Job drawing, mm, ordinate dimensions from the low corner. One solid piece. A direction names the side the tool comes from. Coordinates: 2 decimals unless noted, no trailing zeros. Order: outer loops, then holes, each group sorted by start corner. A loop starts at its lowest first (then second) coordinate and runs counter-clockwise, first axis right, second up. Notation, with made-up numbers: (-33, -11) -> (-16, -11) arc R26 ccw to (-16, 24) -> close; hole circle Ø10 at (-8.75, 29.5). An arc over 180 degrees is marked (long way). Use CSV: the item, a comma, the result in double quotes. Start each with the question number.
(1) Pin check, flat tips, straight feed: pin 1 Ø2 at (x, z) = (8, 4) entering from +Y; pin 2 Ø4 at (x, y) = (6, 11) entering from +Z. Stop position of each tip, or through.
(2) Cut at D-D on y = 3.25. Write the cut outline in (x, z).
(3) Cut at B-B on y = 6.35. Write the cut outline in (x, z).
(4) Probe L1, parallel to Z at x = 5, y = 6.35; L2, parallel to Y at x = 2.75, z = 2.25; L3, parallel to Z at x = 6, y = 1.75. List the from-to ranges inside material, lowest first.
(5) Pull direction Z, two halves, no side cores. Call the marked faces 6, 7 and 8: pulls with the +Z half, pulls with the -Z half, needs draft (parallel to the pull), parting line crosses it, or undercut.
(6) Cut at C-C on z = 1.9. Write the cut outline in (x, y), plus the area to 3 significant figures.
(7) Tool access for the marked faces 1, 2, 3, 4 and 5: list every direction of +Z, -Z, +X, -X, +Y, -Y with a clear straight run to the whole face (end or side of a thin tool).
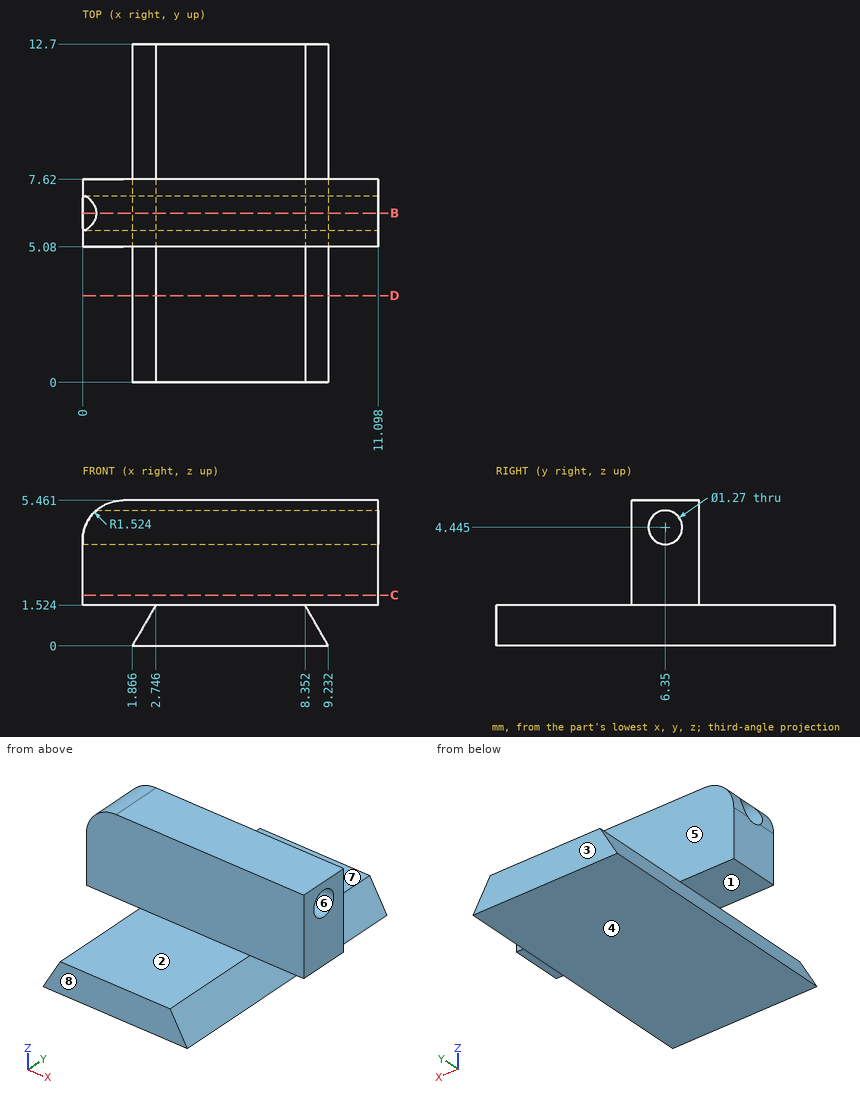
Outcome:
1,pin 1,"y = 7.62"
1,pin 2,"z = 1.52"
2,outline,"(1.87, 0) -> (9.23, 0) -> (8.35, 1.52) -> (2.75, 1.52) -> close"
3,outline,"(0, 1.52) -> (2.75, 1.52) -> (1.87, 0) -> (9.23, 0) -> (8.35, 1.52) -> (11.1, 1.52) -> (11.1, 3.81) -> (0, 3.81) -> close; (0.52, 5.08) -> (11.1, 5.08) -> (11.1, 5.46) -> (1.52, 5.46) arc R1.52 ccw to start"
4,L1,"0 to 3.81, 5.08 to 5.46"
4,L2,"5.08 to 7.62"
4,L3,"0 to 1.52"
5,face 6,"undercut"
5,face 7,"pulls with the +Z half"
5,face 8,"needs draft"
6,outline,"(0, 5.08) -> (11.1, 5.08) -> (11.1, 7.62) -> (0, 7.62) -> close"
6,area,"28.2 mm2"
7,face 1,"-X, +Y, -Y"
7,face 2,"+Z, +X, -X, -Y"
7,face 3,"+Z, -Z, +X, -X, +Y"
7,face 4,"-Z, +X, -X, +Y, -Y"
7,face 5,"+Z, +X, -X, +Y"
